The model under review builds one solid part; all positions refer to its coordinate system, in mm. A direction names the side the tool comes from. Coordinates: 2 decimals unless noted, no trailing zeros. Order: outer loops, then holes, each group sorted by start corner. A loop starts at its lowest first (then second) coordinate and runs counter-clockwise, first axis right, second up. Notation, with made-up numbers: (40.5, 35) -> (44.5, 35) arc R22 ccw to (44.5, 74) -> close; hole circle Ø3 at (34, -13). An arc over 180 degrees is marked (long way). Use one line per item in the form item = value.
Autodesk Inventor part; units mm, degrees
ref_plane "YZ Plane" through (0, 0, 0) normal (1, 0, 0) x (0, 1, 0)
ref_plane "XZ Plane" through (0, 0, 0) normal (0, 1, 0) x (-1, 0, 0)
ref_plane "XY Plane" through (0, 0, 0) normal (0, 0, 1) x (1, 0, 0)
sketch "Sketch1" plane through (0, 0, 0) normal (0, 0, 1) x (1, 0, 0)
  line L0 (-496.5, -135) -> (496.5, -135)
  line L1 (496.5, -135) -> (496.5, 135)
  line L2 (496.5, 135) -> (-496.5, 135)
  line L3 (-496.5, 135) -> (-496.5, -135)
  line L4 (-496.5, -135) -> (496.5, 135) construction
  line L5 (496.5, -135) -> (-496.5, 135) construction
  point P0 (0, 0)
  dimension "d0" = 993
  dimension "d1" = 270
extrude "Plate1" add sketch "Sketch1" along normal blind 0.5
sketch "Sketch2" plane through (496.5, 134.5, 0.5) normal (0, 1, 0) x (-1, 0, 0)
  line L0 (993, 0) -> (0, 0)
  line L1 (0, 0) -> (0, -25)
  line L2 (0, -25) -> (993, -25)
  line L3 (993, -25) -> (993, 0)
edge flange "Flange1" height 25 angle 90 thickness 0.5 bend radius 0.5 thickness toward (0, 1, 0) relief tear relief width 0.5 relief depth 0.25 corner gap 0.5 corner form 0 edges at (0, 135, 0) (0, -135, 0) wall of the first edge with corners at (-496.5, 134.5, 0.5) (496.5, 134.5, 0.5) (496.5, 134.5, -24.5) (-496.5, 134.5, -24.5)
bend "Bend1"
corner "Corner1"
equation "\"d2\" = Thickness"
equation "\"d3\" = BendReliefWidth"
equation "\"d4\" = BendReliefDepth"
equation "\"d5\" = MinimumRemnant"
equation "\"d6\" = TransitionRadius"
equation "\"d9\" = BendRadius"
equation "\"d10\" = CornerReliefSize"
equation "\"d11\" = GapSize"
equation "\"d12\" = JacobiRadiusSize"
equation "\"BendRadius\" = Thickness"
equation "\"BendReliefWidth\" = Thickness"
equation "\"BendReliefDepth\" = 0.5 * Thickness"
equation "\"CornerReliefSize\" = 4 * Thickness"
equation "\"MinimumRemnant\" = 2 * Thickness"
equation "\"TransitionRadius\" = BendRadius"
equation "\"JacobiRadiusSize\" = BendRadius"
equation "\"GapSize\" = Thickness"
equation "\"Space5\" = 0"
equation "\"Space6\" = 0"
equation "\"Space7\" = 0"
properties part number "Acoplador_de_Cuentas"
Item 1: Tool access review of faces 5 (the face through (7, 134.5, -12)), 6 (the face through (-7, 2, 0.5)): name each direction out of +Z, -Z, +X, -X, +Y, -Y from which nothing blocks a thin tool from reaching the whole face with its end or side.
Results found:
face_5 = -Z, +X, -X
face_6 = +Z, +X, -X, +Y, -Y
Item 2: We need section C-C (y = -52). Write out the cut boundary in (x, z), plus the area to 4 significant figures.
Results found:
outline = (-496.5, 0) -> (496.5, 0) -> (496.5, 0.5) -> (-496.5, 0.5) -> close
area = 496.5 mm²
Item 3: We need section A-A (z = -10.75). Write out the cut boundary in (x, y).
Results found:
outline = (-496.5, -135) -> (496.5, -135) -> (496.5, -134.5) -> (-496.5, -134.5) -> close; (-496.5, 134.5) -> (496.5, 134.5) -> (496.5, 135) -> (-496.5, 135) -> close
Item 4: Clearance check with a flat-ended pin moving along its axis: pin 1 (8 mm diameter, centred on x = 380.5, y = 85.5, fed in from -Z). State where the tip first meets the part, or that it passes through.
Results found:
pin_1 = 0
Item 5: Draft analysis for pull direction Y (two halves, no side actions). For faces 1 (the face through (-7, 2, 0)), 2 (the face through (-7, -135, -13)), 3 (the face through (-7, -134.5, -12)), 4 (the face through (7, 135, -13)), state which applies: released by +Y, released by -Y, zero draft, split by the parting line, or undercut.
Results found:
face_1 = undercut
face_2 = released by -Y
face_3 = undercut
face_4 = released by +Y
Item 6: To check wall thickness, follow L1, parallel to Y at x = 183.5, z = -14.5; L2, parallel to Z at x = -259.5, y = -7; L3, parallel to Y at x = 397, z = -0.25. State the ranges of each line that lie inside material, in increasing order. Write a range as from..to.
Results found:
L1 = -135..-134.5, 134.5..135
L2 = 0..0.5
L3 = -134.97..-134.43, 134.43..134.97
Item 7: We need section B-B (x = 356). Write out the cut boundary in (y, z).
Results found:
outline = (-135, -24.5) -> (-134.5, -24.5) -> (-134.5, -0.5) arc R0.5 cw to (-134, 0) -> (134, 0) arc R0.5 cw to (134.5, -0.5) -> (134.5, -24.5) -> (135, -24.5) -> (135, -0.5) arc R1 ccw to (134, 0.5) -> (-134, 0.5) arc R1 ccw to (-135, -0.5) -> close
